Design review of the part shown in the three views and the two pictorial views. Dimensions are in mm from the part's minimum x, y and z. A direction names the side the tool comes from. Give positions to 0.01 mm unless a question says otherwise; leave off trailing zeros. Loops run counter-clockwise (first coordinate to the right, second up) from the corner with the lowest first, then second, coordinate; pieces in that order, holes last. Notation, with made-up numbers: (87, 87.25) -> (113, 87.25) arc R20 ccw to (113, 97.25) -> close; hole circle Ø11 at (62.25, 24). An arc over 180 degrees is marked (long way). Use CSV: the item, a comma, the result in double quotes. Start each with the question number.
Item 1: We need section C-C (y = 38). State the section outline as (x, z) points.
Item 2: For the marked faces 1, 2 and 3, list the 3-axis set-ups (+Z, -Z, +X, -X, +Y, -Y) from which the entire face can be reached by the end or side of a thin tool; tool diameter is ignored.
Item 3: Clearance check with flat-ended pins moving along their axes: pin 1 (12.5 mm diameter, centred on x = 21, y = 28.5, fed in from +Z); pin 2 (12 mm diameter, centred on x = 25.5, z = 26.5, fed in from -Y); pin 3 (2 mm diameter, centred on x = 24.5, z = 1, fed in from -Y) (1 decimal); pin 4 (1.5 mm diameter, centred on y = 37.5, z = 16.5, fed in from -X). State where each tip first meets the part, or that it passes through.
Item 4: The part is to be moulded in two halves that separate along Y. For the marked faces 4, 5 and 6, say which applies: +Y half, -Y half, draft (parallel to the pull), parting line (faces both ways), or undercut.
Item 5: Wall thickness on line 1 along Y through (x, z) = (21, 22); line 2 along Z through (x, y) = (30.5, 38); line 3 along Y through (x, z) = (21, 12): over which ranges is each line inside the solid? List them lowest first. Write a range as from..to.
Item 6: We need section D-D (x = 12.5). State the section outline as (y, z) points.
Item 7: We need section A-A (x = 5). State the section outline as (y, z) points.
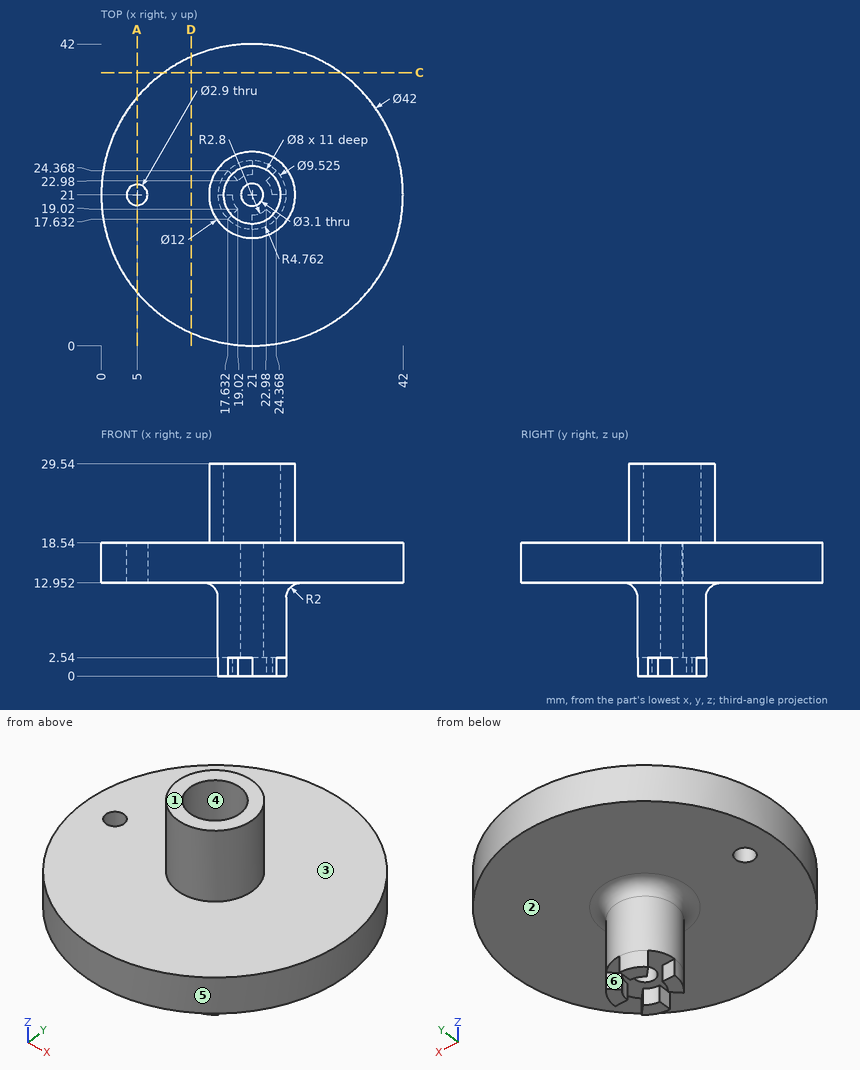
Results found:
1,outline,"(8.67, 12.95) -> (33.33, 12.95) -> (33.33, 18.54) -> (8.67, 18.54) -> close"
2,face 1,"+Z, +X, -X, +Y, -Y"
2,face 2,"-Z"
2,face 3,"+Z"
3,pin 1,"z = 29.54"
3,pin 2,"y = 15"
3,pin 3,"y = 16.9"
3,pin 4,"x = 7.11"
4,face 4,"undercut"
4,face 5,"parting line"
4,face 6,"+Y half"
5,line 1,"15..17, 25..27"
5,line 2,"12.95..18.54"
5,line 3,"15.94..19.45, 22.55..26.06"
6,outline,"(1.8, 12.95) -> (40.2, 12.95) -> (40.2, 18.54) -> (1.8, 18.54) -> close"
7,outline,"(7.4, 12.95) -> (19.55, 12.95) -> (19.55, 18.54) -> (7.4, 18.54) -> close; (22.45, 12.95) -> (34.6, 12.95) -> (34.6, 18.54) -> (22.45, 18.54) -> close"
